Source: CAD feature listing. Evaluate the final solid. Frame: model axes, mm. Face numbers are marked on the shaded views. A direction names the side the tool comes from. Coordinates: 2 decimals unless noted, no trailing zeros. Loops run counter-clockwise (first coordinate to the right, second up) from the corner with the lowest first, then second, coordinate; pieces in that order, holes last.
Autodesk Inventor part; units mm, degrees
ref_plane "Work Plane1" through (6.228, -54, -6.35) normal (0, 0, -1) x (0, 1, 0)
ref_plane "YZ Plane" through (0, 0, 0) normal (1, 0, 0) x (0, 1, 0)
ref_plane "XZ Plane" through (0, 0, 0) normal (0, 1, 0) x (-1, 0, 0)
sketch "Sketch1" plane through (0, 0, 0) normal (0, 0, 1) x (1, 0, 0)
  line L0 (-2.81, 5) -> (2.81, 5)
  line L1 (2.81, 5) -> (2.81, -33.1)
  line L2 (2.81, -33.1) -> (-2.81, -33.1)
  line L3 (-2.81, -33.1) -> (-2.81, 5)
  line L4 (-2.81, -33.1) -> (-8.43, -33.1)
  line L5 (-8.43, -33.1) -> (-8.43, -7.2065)
  line L6 (-8.43, -7.2065) -> (-2.81, -7.2065)
  line L7 (-2.81, -7.2065) -> (-2.81, -33.1)
  line L8 (-13.3844, -4.6707) -> (3.9886, -4.5258) construction
  line L9 (4.1365, -22.2635) -> (-13.2364, -22.4084) construction
  line L10 (-18.4107, -1.5425) -> (-18.3842, -4.7124) construction
  line L11 (42.6603, -9.7914) -> (42.6338, -6.6215)
  line L12 (0, -40.72) -> (0, 12.62) construction
  line L13 (2.81, -33.1) -> (8.43, -33.1)
  line L14 (8.43, -33.1) -> (8.43, -7.2065)
  line L15 (8.43, -7.2065) -> (2.81, -7.2065)
  line L16 (2.81, -7.2065) -> (2.81, -33.1)
  point P0 (0, 0)
  point P1 (42.647, -8.2065)
  dimension "d0" = 1
  dimension "d1" = 1
  dimension "d2" = 1
  dimension "d3" = 38.1
  dimension "d4" = 1
ref_plane "Work Plane1" through (6.228, -54, -6.35) normal (0, 0, -1) x (0, 1, 0)
extrude "Extrusion1" add sketch "Sketch1" along normal mid plane 12.7
properties part number "ForearmActuatorConnectorBoundingBox"
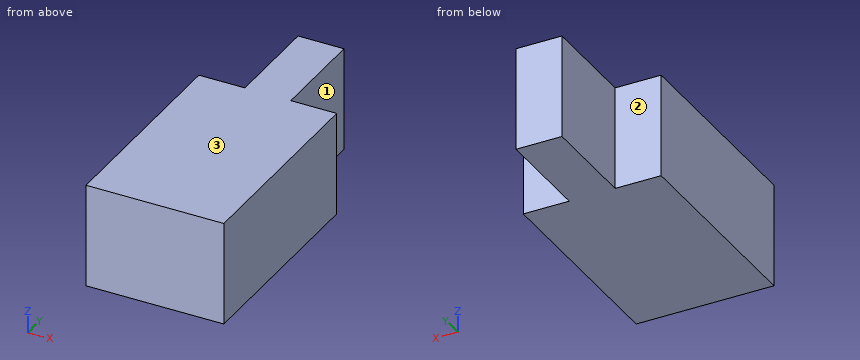
Q1. Material intervals for line 1 along X through (y, z) = (-1.5, 5.75); line 2 along Y through (x, z) = (3.25, -1.5), sorted ascending.
Q2. Section query C-C on x = -5. Return the cut outline in (y, z).
Q3. First-contact query: pin 1 Ø1.7 at (x, z) = (-5.5, 2) entering from +Y; pin 2 Ø6 at (y, z) = (-1, 0) entering from +X. Flat tips, straight axial feed; report the tip coordinate or a pass-through.
Q4. Section query A-A on z = 5.25. Return the cut outline in (x, y), then the cut area to 3 significant figures.
Q5. Section query B-B on y = -3. Return the cut outline in (x, z), then the cut area to 3 significant figures.
Q6. Reachability of the marked faces 1, 2 and 3 from +Z, -Z, +X, -X, +Y, -Y: full face, straight path, thin tool, end or side. Return the list, or none.
Resolved:
1. line 1: x = -2.81 to 2.81
1. line 2: y = -33.1 to -7.21
2. outline: (-33.1, -6.35) - (-7.21, -6.35) - (-7.21, 6.35) - (-33.1, 6.35) - close
3. pin 1: stops at y = -7.21
3. pin 2: stops at x = 2.81
4. outline: (-8.43, -33.1) - (8.43, -33.1) - (8.43, -7.21) - (2.81, -7.21) - (2.81, 5) - (-2.81, 5) - (-2.81, -7.21) - (-8.43, -7.21) - close
4. area: 505 mm2
5. outline: (-2.81, -6.35) - (2.81, -6.35) - (2.81, 6.35) - (-2.81, 6.35) - close
5. area: 71.4 mm2
6. face 1: +Z, -Z, +X, +Y
6. face 2: +Z, -Z, -X, +Y
6. face 3: +Z, +X, -X, +Y, -Y
